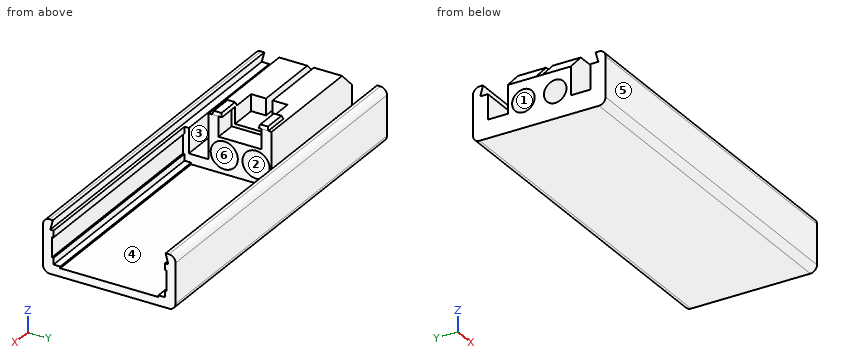
```python
from build123d import *

# Parameters (mm, degrees)
SKETCH_W        = 105
SKETCH_H        = 40
PAD_DEPTH       = 16
SKETCH001_W     = 65
SKETCH001_H     = 33.6
POCKET_DEPTH    = 13
SKETCH002_R     = 3.4
POCKET001_DEPTH = 40.001
SKETCH014_R     = 4.1
POCKET002_DEPTH = 25
SKETCH006_W     = 40
SKETCH006_H     = 6
POCKET003_DEPTH = 10.5
SKETCH011_W     = 105
SKETCH011_H     = 34
POCKET004_DEPTH = 3
POCKET004_TAPER = -15
SKETCH008_W     = 65
SKETCH008_H     = 29.6
POCKET005_DEPTH = 0.5
SKETCH010_W     = 65
SKETCH010_H     = 6
POCKET006_DEPTH = 0.5
SKETCH015_W     = 65
SKETCH015_H     = 6
POCKET007_DEPTH = 0.5
SKETCH016_W     = 40
SKETCH016_H     = 19
PAD001_DEPTH    = 6
SKETCH017_W     = 6.5
SKETCH017_H     = 13
POCKET008_DEPTH = 6
SKETCH018_W     = 8
SKETCH018_H     = 11
POCKET009_DEPTH = 5
SKETCH019_W     = 25.5
SKETCH019_H     = 2
POCKET010_DEPTH = 5
SKETCH020_W     = 7.5
SKETCH020_H     = 3
PAD002_DEPTH    = 1
PAD002_TAPER    = 20
FILLET_R        = 2
CHAMFER_SIZE    = 5


with BuildPart() as part:
    # Sketch → Pad (new body)
    with BuildSketch(Plane.XY):
        Rectangle(SKETCH_W, SKETCH_H)
    extrude(amount=PAD_DEPTH)

    # Sketch001 (on Face6 of Pad) → Pocket (cut)
    with BuildSketch(Plane.XY.offset(16)):
        with Locations((20, 0)):
            Rectangle(SKETCH001_W, SKETCH001_H)
    extrude(amount=-POCKET_DEPTH, mode=Mode.SUBTRACT)

    # Sketch002 (on Face10 of Pocket) → Pocket001 (cut, through all)
    with BuildSketch(Plane.YZ.offset(-12.5)):
        with Locations((4.8, 8)):
            Circle(SKETCH002_R)
        with Locations((-4.8, 8)):
            Circle(SKETCH002_R)
    extrude(amount=-POCKET001_DEPTH, mode=Mode.SUBTRACT)

    # Sketch014 (on Face12 of Pocket001) → Pocket002 (cut)
    with BuildSketch(Plane.YZ.offset(-12.5)):
        with Locations((4.8, 8)):
            Circle(SKETCH014_R)
        with Locations((-4.8, 8)):
            Circle(SKETCH014_R)
    extrude(amount=-POCKET002_DEPTH, mode=Mode.SUBTRACT)

    # Sketch006 → Pocket003 (cut)
    with BuildSketch(Plane.XY.offset(16)):
        with Locations((-32.5, 12.5)):
            Rectangle(SKETCH006_W, SKETCH006_H)
        with Locations((-32.5, -12.5)):
            Rectangle(SKETCH006_W, SKETCH006_H)
    extrude(amount=-POCKET003_DEPTH, mode=Mode.SUBTRACT)

    # Sketch011 → Pocket004 (cut)
    with BuildSketch(Plane.XY.offset(16)):
        Rectangle(SKETCH011_W, SKETCH011_H)
    extrude(amount=-POCKET004_DEPTH, taper=POCKET004_TAPER, mode=Mode.SUBTRACT)

    # Sketch008 → Pocket005 (cut)
    with BuildSketch(Plane.XY.offset(3)):
        with Locations((20, 0)):
            Rectangle(SKETCH008_W, SKETCH008_H)
    extrude(amount=-POCKET005_DEPTH, mode=Mode.SUBTRACT)

    # Sketch010 → Pocket006 (cut)
    with BuildSketch(Plane(origin=(0, -16.8, 0), x_dir=(-1, 0, 0), z_dir=(0, 1, 0))):
        with Locations((-20, 8)):
            Rectangle(SKETCH010_W, SKETCH010_H)
    extrude(amount=-POCKET006_DEPTH, mode=Mode.SUBTRACT)

    # Sketch015 (on Face31 of Pocket006) → Pocket007 (cut)
    with BuildSketch(Plane.XZ.offset(-16.8)):
        with Locations((20, 8)):
            Rectangle(SKETCH015_W, SKETCH015_H)
    extrude(amount=-POCKET007_DEPTH, mode=Mode.SUBTRACT)

    # Sketch016 (on Face11 of Pocket007) → Pad001 (join)
    with BuildSketch(Plane.XY.offset(13)):
        with Locations((-32.5, 0)):
            Rectangle(SKETCH016_W, SKETCH016_H)
    extrude(amount=PAD001_DEPTH)

    # Sketch017 (on Face39 of Pad001) → Pocket008 (cut)
    with BuildSketch(Plane.XY.offset(19)):
        with Locations((-15.75, 0)):
            Rectangle(SKETCH017_W, SKETCH017_H)
    extrude(amount=-POCKET008_DEPTH, mode=Mode.SUBTRACT)

    # Sketch018 (on Face39 of Pocket008) → Pocket009 (cut)
    with BuildSketch(Plane.XY.offset(19)):
        with Locations((-23, 0)):
            Rectangle(SKETCH018_W, SKETCH018_H)
    extrude(amount=-POCKET009_DEPTH, mode=Mode.SUBTRACT)

    # Sketch019 (on Face39 of Pocket009) → Pocket010 (cut)
    with BuildSketch(Plane.XY.offset(19)):
        with Locations((-39.75, 0)):
            Rectangle(SKETCH019_W, SKETCH019_H)
    extrude(amount=-POCKET010_DEPTH, mode=Mode.SUBTRACT)

    # Sketch020 (on Face42 of Pocket010) → Pad002 (join)
    with BuildSketch(Plane.XY.offset(19)):
        with Locations((-16.25, 7)):
            Rectangle(SKETCH020_W, SKETCH020_H)
        with Locations((-16.25, -7)):
            Rectangle(SKETCH020_W, SKETCH020_H)
    extrude(amount=PAD002_DEPTH, taper=PAD002_TAPER)

    # Fillet
    fillet_edges = [part.edges().sort_by_distance(p)[0] for p in [
        (0, -20, 16),
        (0, -20, 0),
        (0, 20, 16),
        (0, 20, 0),
    ]]
    fillet(fillet_edges, radius=FILLET_R)

    # Chamfer
    chamfer_edges = [part.edges().sort_by_distance(p)[0] for p in [
        (-52.5, -5.25, 19),
        (-52.5, 5.25, 19),
    ]]
    chamfer(chamfer_edges, length=CHAMFER_SIZE)


solid = part.part
```
Check sheet for the modelled part. Datum: model origin and axes. Units: mm. Face numbers are marked on the shaded views. A direction names the side the tool comes from. Give positions to 0.01 mm unless a question says otherwise; leave off trailing zeros. Order: outer loops, then holes, each group sorted by start corner. A loop starts at its lowest first (then second) coordinate and runs counter-clockwise, first axis right, second up. Notation, with made-up numbers: (-23, 70) -> (10, 70) arc R24 ccw to (10, 96) -> close; hole circle Ø7 at (40.25, 9.25). An arc over 180 degrees is marked (long way). Return JSON: item names as keys, results as strings.
1. Cross-section at B-B, the plane y = -11. Record the cut outline in (x, z).
From the geometry:
{"outline": "(-52.5, 0) -> (52.5, 0) -> (52.5, 2.5) -> (-12.5, 2.5) -> (-12.5, 5.5) -> (-52.5, 5.5) -> close"}
2. Material ranges on probe 1 along Z at (x, y) = (-17.75, -4.8); probe 2 along Z at (x, y) = (-47.25, 4.8); probe 3 along Z at (x, y) = (37.5, -10), recorded low to high. Write a range as [from, to].
From the geometry:
{"probe 1": "[0, 3.9], [12.1, 13]", "probe 2": "[0, 4.6], [11.4, 19]", "probe 3": "[0, 2.5]"}
3. Cross-section at A-A, the plane z = 8. Count the separate pieces of the cut face and the enclosed holes in it, plus the area to 3 significant figures.
From the geometry:
{"separate pieces": "5", "enclosed holes": "0", "area": "857 mm^2"}
4. Mould release check, pull along Z, two halves, no side actions. Record for the marked faces 4, 5 and 6: +Z half, -Z half, draft (parallel to the pull), parting line (faces both ways), or undercut.
From the geometry:
{"face 4": "+Z half", "face 5": "draft", "face 6": "undercut"}
5. Set-up check for the marked faces 1, 2 and 3: record each of +Z, -Z, +X, -X, +Y, -Y from which the full face is reachable in a straight line by a thin tool's end or side.
From the geometry:
{"face 1": "+X, -X", "face 2": "+X", "face 3": "+Z, +X, -X"}
6. Go/stop test with flat-tipped pins: P1, Ø7, axis at x = -15, y = -1.5, coming from the +Z side; P2, Ø15, axis at x = 15.5, y = -5.5, coming from the +Z side; P3, Ø5, axis at y = -3.5, z = 16, coming from the +X side. Record where each tip stops, or that it passes through.
From the geometry:
{"P1": "z = 13", "P2": "z = 2.5", "P3": "x = -19"}
